```python
from build123d import *

# Parameters (mm, degrees)
F0_W           = 3
F0_H           = 4.5
F3_D           = 5.5
F3_CBORE_D     = 9
F3_CBORE_DEPTH = 7


with BuildPart() as f1:
    # F0 (on Front) → F1 (revolve)
    with BuildSketch(Plane.XZ):
        Polygon((-71.96031, 2.75), (-71.96031, 0), (-67.96031, 0), (-67.96031, 4.5), (-71.96031, 4.5), align=None)
        Polygon((-67.96031, 8), (-67.96031, 4.5), (-64.96031, 4.5), (-64.96031, 6.267949), align=None)
        with Locations((-66.46031, 2.25)):
            Rectangle(F0_W, F0_H)
        Polygon((-112.46031, 0), (-109.96031, 0), (-109.96031, 2.75), (-109.96031, 5), (-112.46031, 5), align=None)
        Polygon((-109.96031, 2.75), (-71.96031, 2.75), (-71.96031, 4.5), (-67.96031, 4.5), (-67.96031, 8), (-109.96031, 8), (-109.96031, 5), align=None)
        Polygon((-112.96031, 0), (-112.46031, 0), (-112.46031, 5), (-112.96031, 4.5), align=None)
        Polygon((-81.96031, 0), (-71.96031, 0), (-71.96031, 2.75), (-109.96031, 2.75), (-109.96031, 0), align=None)
    revolve(axis=Axis((-88.96031, 0, 0), (-1, 0, 0)))

    # F3 (through all)
    with Locations(Plane.YZ.offset(-64.96031)):
        with Locations((0, 0)):
            CounterBoreHole(F3_D / 2, F3_CBORE_D / 2, F3_CBORE_DEPTH)


solid = f1.part
```
The listing builds one solid part. Answer for the finished solid, in the listing's coordinates (mm). A direction names the side the tool comes from. Coordinates: 2 decimals unless noted, no trailing zeros. Write each loop counter-clockwise with the first axis right and the second up, starting at its lowest first coordinate (ties: lowest second). Pieces come first, ordered by that corner, then holes.
Q1. Which of the six approach directions +Z, -Z, +X, -X, +Y, -Y give full straight-line access (tool end or side, diameter ignored) to faces 4 (the cylindrical face through (-111.23, -4.88, -1.08)), 5 (the cylindrical face through (-92.747, 0.596, -2.685)), 6 (the flat face through (-71.96, 0, -3))?
Returned:
face 4: -X
face 5: +X, -X
face 6: +X
Q2. Find the intervals of material crossed by line 1 along X through (y, z) = (2.25, -2.5); line 2 along X through (y, z) = (5, -2); line 3 along Y through (x, z) = (-88.5, -2), in increasing order.
Returned:
line 1: x = -112.96 to -71.96
line 2: x = -109.96 to -64.96
line 3: y = -7.75 to -1.89, 1.89 to 7.75
Q3. The mould has two halves that part along Y. Classify faces 1 (the conical face through (-65.148, -6.225, -1.382)), 2 (the cylindrical face through (-68.41, -0.59, 4.46)), 3 (the flat face through (-112.96, -3, 0)): released by +Y, released by -Y, zero draft, split by the parting line, or undercut.
Returned:
face 1: split by the parting line
face 2: undercut
face 3: zero draft
Q4. Section A-A, the plane y = 0 is taken. Write down the section's boundary in (x, z), then the cut area to 3 significant figures.
Returned:
outline: (-112.96, -4.5) - (-112.46, -5) - (-109.96, -5) - (-109.96, -8) - (-67.96, -8) - (-64.96, -6.27) - (-64.96, -4.5) - (-71.96, -4.5) - (-71.96, -2.75) - (-112.96, -2.75) - close; (-112.96, 2.75) - (-71.96, 2.75) - (-71.96, 4.5) - (-64.96, 4.5) - (-64.96, 6.27) - (-67.96, 8) - (-109.96, 8) - (-109.96, 5) - (-112.46, 5) - (-112.96, 4.5) - close
area: 456 mm2
Q5. Section C-C, the plane x = -108 is taken. Write down the section's boundary in (y, z).
Returned:
outline: circle Ø16 at (0, 0); hole circle Ø5.5 at (0, 0)
Q6. Given P1, Ø2, axis at x = -91, z = -4, coming from the -Y side; P2, Ø5, axis at x = -98.5, z = 4, coming from the +Y side; P3, Ø1, axis at x = -97.5, z = 2.5, coming from the +Y side; P4, Ø5, axis at y = 0, z = 0, coming from the +X side, each flat-ended and moving along its own axis, determine where each tip first touches the part or whether it passes through.
Returned:
P1: stops at y = -7.42
P2: stops at y = 7.86
P3: stops at y = 7.75
P4: passes through
